Can you work these out from the drawing? Everything is in mm from the part's minimum corner. Give positions to 0.01 mm unless a question says otherwise; leave off trailing zeros. Loops run counter-clockwise (first coordinate to the right, second up) from the corner with the lowest first, then second, coordinate; pieces in that order, holes last.
Q1. If we section it at A-A (y = 30): Please give me the cut outline in (x, z), plus the area to 3 significant figures.
Q2. Will these pins go through, and if not, where does the flat tip stop? P1, Ø5, axis at y = 10.5, z = 61.5, coming from the +X side; P2, Ø1.5, axis at y = 6.5, z = 60, coming from the -X side; P3, Ø12, axis at y = 42, z = 23.5, coming from the +X side.
Q3. I need wall thicknesses on line 1 (X direction, y = 31, z = 33); line 2 (Z direction, x = 41.5, y = 51.5); line 3 (Y direction, x = 51, z = 63). Which ranges of each line are inside material? Lowest first, please.
Q4. If we section it at C-C (z = 53): Please give me the cut outline in (x, y).
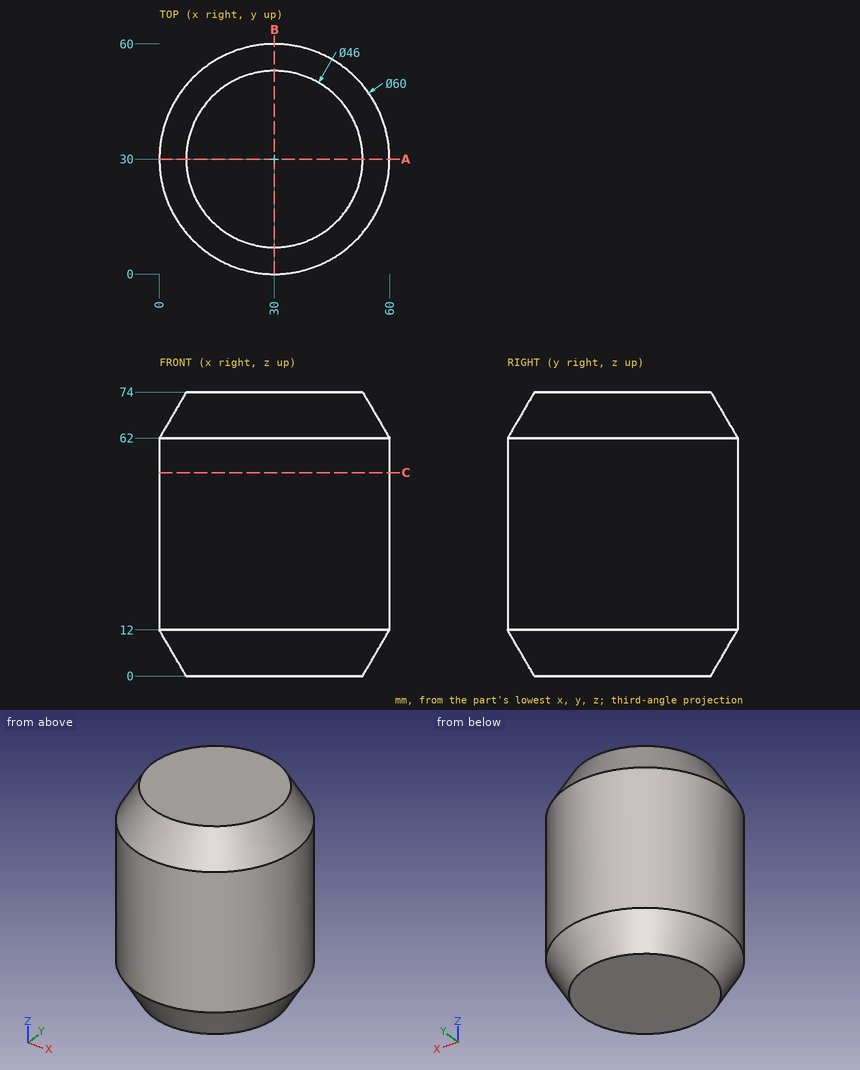
Check sheet entries:
1. outline: (0, 12) - (7, 0) - (53, 0) - (60, 12) - (60, 62) - (53, 74) - (7, 74) - (0, 62) - close
1. area: 4,270 mm2
2. P1: stops at x = 54.72
2. P2: stops at x = 10.44
2. P3: stops at x = 59.39
3. line 1: x = 0.02 to 59.98
3. line 2: z = 2.37 to 71.63
3. line 3: y = 9.4 to 50.6
4. outline: circle Ø60 at (30, 30)
